```python
from build123d import *

# Parameters (mm, degrees)
SKETCH1_R           = 12.6
BOSS_EXTRUDE1_DEPTH = 19
SKETCH2_R           = 12.1
BOSS_EXTRUDE2_DEPTH = 30
SKETCH3_R           = 12.1
SKETCH3_R_2         = 11.75
BOSS_EXTRUDE3_DEPTH = 1
SKETCH4_R           = 3.2
BOSS_EXTRUDE4_DEPTH = 2.3
FILLET1_R           = 1
BOSS_EXTRUDE5_DEPTH = 0.2
SKETCH6_R           = 0.5
CUT_EXTRUDE1_DEPTH  = 20
CUT_EXTRUDE2_DEPTH  = 0.1
CIRPATTERN1_COUNT   = 4
SKETCH8_R           = 3.5
BOSS_EXTRUDE6_DEPTH = 2.5
SKETCH9_R           = 2
BOSS_EXTRUDE7_DEPTH = 12
CUT_EXTRUDE3_START  = -10
CUT_EXTRUDE3_DEPTH  = 10
SKETCH11_R          = 1.5
CUT_EXTRUDE4_DEPTH  = 10


with BuildPart() as part:
    # Sketch1 → Boss-Extrude1 (new body)
    with BuildSketch(Plane.XY):
        Circle(SKETCH1_R)
    extrude(amount=BOSS_EXTRUDE1_DEPTH)

    # Sketch2 → Boss-Extrude2 (add)
    with BuildSketch(Plane.XY.offset(19)):
        Circle(SKETCH2_R)
    extrude(amount=BOSS_EXTRUDE2_DEPTH)

    # Sketch3 → Boss-Extrude3 (add)
    with BuildSketch(Plane.XY.offset(49)):
        Circle(SKETCH3_R)
        Circle(SKETCH3_R_2, mode=Mode.SUBTRACT)
    extrude(amount=BOSS_EXTRUDE3_DEPTH)

    # Sketch4 → Boss-Extrude4 (add)
    with BuildSketch(Plane.XY.offset(49)):
        Circle(SKETCH4_R)
    extrude(amount=BOSS_EXTRUDE4_DEPTH)

    # Fillet1
    fillet1_edges = [part.edges().sort_by_distance(p)[0] for p in [
        (-3.2, 0, 51.3),
    ]]
    fillet(fillet1_edges, radius=FILLET1_R)

    # Sketch5 → Boss-Extrude5 (add)
    with BuildSketch(Plane.XY.offset(49)):
        with BuildLine():
            Line((-7.8, 2), (-7.8, -2))
            ThreePointArc((-7.8, -2), (-9, -3.2), (-10.2, -2))
            Line((-10.2, -2), (-10.2, 2))
            ThreePointArc((-10.2, 2), (-9, 3.2), (-7.8, 2))
        make_face()
        with BuildLine():
            Line((10.2, 2.236300976), (10.2, -2.236300976))
            ThreePointArc((10.2, -2.236300976), (9, -3.436300976), (7.8, -2.236300976))
            Line((7.8, -2.236300976), (7.8, 2.236300976))
            ThreePointArc((7.8, 2.236300976), (9, 3.436300976), (10.2, 2.236300976))
        make_face()
    extrude(amount=BOSS_EXTRUDE5_DEPTH)

    # Sketch6 → Cut-Extrude1 (cut)
    with BuildSketch(Plane.XY.offset(49)):
        with Locations((-3.815326444, 3.815326444)):
            Circle(SKETCH6_R)
        with Locations((3.815326444, -4.184114524)):
            Circle(SKETCH6_R)
        with BuildLine():
            Line((-2.763844704, 3.00518783), (-2.64955067, 2.880913468))
            ThreePointArc((-2.64955067, 2.880913468), (-2.623197255, 2.81031672), (-2.653603933, 2.741368644))
            ThreePointArc((-2.653603933, 2.741368644), (-3.815326444, 0), (-2.653603933, -2.741368644))
            ThreePointArc((-2.653603933, -2.741368644), (-2.623197255, -2.81031672), (-2.64955067, -2.880913468))
            Line((-2.64955067, -2.880913468), (-2.763844704, -3.00518783))
            ThreePointArc((-2.763844704, -3.00518783), (-2.834492952, -3.037450785), (-2.906924389, -3.00941937))
            ThreePointArc((-2.906924389, -3.00941937), (-4.184114524, 0), (-2.906924389, 3.00941937))
            ThreePointArc((-2.906924389, 3.00941937), (-2.834492952, 3.037450785), (-2.763844704, 3.00518783))
        make_face()
        with BuildLine():
            Line((2.64955067, 2.880913468), (2.763844704, 3.00518783))
            ThreePointArc((2.763844704, 3.00518783), (2.834492952, 3.037450785), (2.906924389, 3.00941937))
            ThreePointArc((2.906924389, 3.00941937), (4.184114524, 0), (2.906924389, -3.00941937))
            ThreePointArc((2.906924389, -3.00941937), (2.834492952, -3.037450785), (2.763844704, -3.00518783))
            Line((2.763844704, -3.00518783), (2.64955067, -2.880913468))
            ThreePointArc((2.64955067, -2.880913468), (2.623197255, -2.81031672), (2.653603933, -2.741368644))
            ThreePointArc((2.653603933, -2.741368644), (3.815326444, 0), (2.653603933, 2.741368644))
            ThreePointArc((2.653603933, 2.741368644), (2.623197255, 2.81031672), (2.64955067, 2.880913468))
        make_face()
    extrude(amount=-CUT_EXTRUDE1_DEPTH, mode=Mode.SUBTRACT)

    # Sketch7 → Cut-Extrude2 (cut)
    with BuildSketch(Plane(origin=(0, 0, 0), x_dir=(-1, 0, 0), z_dir=(0, 0, -1))):
        with BuildLine():
            Line((4, 10.246950766), (1.709090909, 4.3782426))
            ThreePointArc((1.709090909, 4.3782426), (3.323401872, 3.323401872), (4.3782426, 1.709090909))
            Line((4.3782426, 1.709090909), (10.246950766, 4))
            ThreePointArc((10.246950766, 4), (7.778174593, 7.778174593), (4, 10.246950766))
        make_face()
    cut_extrude2 = extrude(amount=-CUT_EXTRUDE2_DEPTH, mode=Mode.SUBTRACT)

    # CirPattern1: Cut-Extrude2 ×4 about axis
    cirpattern1_axis = Axis((0, 0, 0), (0, 0, 1))
    for i in range(1, CIRPATTERN1_COUNT):
        add(cut_extrude2.rotate(cirpattern1_axis, i * 360 / CIRPATTERN1_COUNT), mode=Mode.SUBTRACT)

    # Sketch8 → Boss-Extrude6 (add)
    with BuildSketch(Plane(origin=(0, 0, 0), x_dir=(-1, 0, 0), z_dir=(0, 0, -1))):
        Circle(SKETCH8_R)
    extrude(amount=BOSS_EXTRUDE6_DEPTH)

    # Sketch9 → Boss-Extrude7 (add)
    with BuildSketch(Plane(origin=(0, 0, -2.5), x_dir=(-1, 0, 0), z_dir=(0, 0, -1))):
        Circle(SKETCH9_R)
    extrude(amount=BOSS_EXTRUDE7_DEPTH)

    # Sketch10 → Cut-Extrude3 (cut)
    with BuildSketch(Plane(origin=(0, 0, -14.5), x_dir=(-1, 0, 0), z_dir=(0, 0, -1)).offset(CUT_EXTRUDE3_START)):
        with BuildLine():
            Line((-1.322875656, 1.5), (1.322875656, 1.5))
            ThreePointArc((1.322875656, 1.5), (0, 2), (-1.322875656, 1.5))
        make_face()
    extrude(amount=CUT_EXTRUDE3_DEPTH, mode=Mode.SUBTRACT)

    # Sketch11 → Cut-Extrude4 (cut)
    with BuildSketch(Plane(origin=(0, 0, 0), x_dir=(-1, 0, 0), z_dir=(0, 0, -1))):
        with Locations((-8.5, 0)):
            Circle(SKETCH11_R)
        with Locations((8.5, 0)):
            Circle(SKETCH11_R)
    extrude(amount=-CUT_EXTRUDE4_DEPTH, mode=Mode.SUBTRACT)


solid = part.part
```
The listing builds one solid part. Answer for the finished solid, in the listing's coordinates (mm). A direction names the side the tool comes from. Coordinates: 2 decimals unless noted, no trailing zeros. Write each loop counter-clockwise with the first axis right and the second up, starting at its lowest first coordinate (ties: lowest second). Pieces come first, ordered by that corner, then holes.
Q1. Section A-A, the plane z = 32 is taken. Write down the section's boundary in (x, y).
Returned:
outline: circle Ø24.2 at (0, 0); hole circle Ø1 at (-3.82, 3.82); hole (-2.91, -3.01) arc R0.1 ccw to (-2.76, -3.01) - (-2.65, -2.88) arc R0.1 ccw to (-2.65, -2.74) arc R3.82 cw to (-2.65, 2.74) arc R0.1 ccw to (-2.65, 2.88) - (-2.76, 3.01) arc R0.1 ccw to (-2.91, 3.01) arc R4.18 ccw to start; hole (2.65, -2.88) - (2.76, -3.01) arc R0.1 ccw to (2.91, -3.01) arc R4.18 ccw to (2.91, 3.01) arc R0.1 ccw to (2.76, 3.01) - (2.65, 2.88) arc R0.1 ccw to (2.65, 2.74) arc R3.82 cw to (2.65, -2.74) arc R0.1 ccw to start; hole circle Ø1 at (3.82, -4.18)
Q2. Section C-C, the plane y = 5 is taken. Write down the section's boundary in (x, z).
Returned:
outline: (-11.57, 0) - (-9.8, 0) - (-9.8, 0.1) - (-1.95, 0.1) - (-1.95, 0) - (1.95, 0) - (1.95, 0.1) - (9.8, 0.1) - (9.8, 0) - (11.57, 0) - (11.57, 19) - (11.02, 19) - (11.02, 50) - (10.63, 50) - (10.63, 49) - (-10.63, 49) - (-10.63, 50) - (-11.02, 50) - (-11.02, 19) - (-11.57, 19) - close
Q3. Section B-B, the plane x = 0 is taken. Write down the section's boundary in (y, z), then the cut area to 3 significant figures.
Returned:
outline: (-12.6, 0) - (-3.5, 0) - (-3.5, -2.5) - (-2, -2.5) - (-2, -14.5) - (1.5, -14.5) - (1.5, -4.5) - (2, -4.5) - (2, -2.5) - (3.5, -2.5) - (3.5, 0) - (12.6, 0) - (12.6, 19) - (12.1, 19) - (12.1, 50) - (11.75, 50) - (11.75, 49) - (3.2, 49) - (3.2, 50.3) arc R1 ccw to (2.2, 51.3) - (-2.2, 51.3) arc R1 ccw to (-3.2, 50.3) - (-3.2, 49) - (-11.75, 49) - (-11.75, 50) - (-12.1, 50) - (-12.1, 19) - (-12.6, 19) - close
area: 1,280 mm2
Q4. Find the intervals of material crossed by line 1 along Y through (x, z) = (0, 49.5); line 2 along Z through (x, y) = (11, -4.25); line 3 along Z through (x, y) = (5, 9), in increasing order.
Returned:
line 1: y = -12.1 to -11.75, -3.2 to 3.2, 11.75 to 12.1
line 2: z = 0 to 50
line 3: z = 0.1 to 49
Q5. Given P1, Ø6, axis at x = -7.5, y = -2.5, coming from the -Z side; P2, Ø1, axis at y = 8, z = 19, coming from the -X side; P3, Ø1, axis at x = 7, z = 15, coming from the +Y side, each flat-ended and moving along its own axis, determine where each tip first touches the part or whether it passes through.
Returned:
P1: stops at z = 0
P2: stops at x = -10.12
P3: stops at y = 10.79
Q6. The mould has two halves that part along Y. Classify faces 1 (the cylindrical face through (-3.233, -1.341, -1.232)), 2 (the flat face through (-6, -6, 0.1)), 3 (the flat face through (3, -3, 0)): released by +Y, released by -Y, zero draft, split by the parting line, or undercut.
Returned:
face 1: split by the parting line
face 2: undercut
face 3: zero draft
Q7. Which of the six approach directions +Z, -Z, +X, -X, +Y, -Y give full straight-line access (tool end or side, diameter ignored) to faces 4 (the cylindrical face through (0, -2, -8)), 5 (the cylindrical face through (11.18, -4.63, 34.28))?
Returned:
face 4: -Z
face 5: +Z
Q8. Section D-D, the plane z = -7.5 is taken. Write down the section's boundary in (x, y).
Returned:
outline: (-1.32, 1.5) arc R2 ccw (long way) to (1.32, 1.5) - close
